The listing builds one solid part. Answer for the finished solid, in the listing's coordinates (mm). A direction names the side the tool comes from. Give positions to 0.01 mm unless a question says otherwise; leave off trailing zeros. Order: outer loops, then holes, each group sorted by start corner. A loop starts at its lowest first (then second) coordinate and runs counter-clockwise, first axis right, second up. Notation, with made-up numbers: M -33.5,72.5 L 15.5,72.5 A26 cw 15.5,88.5 Z; hole C -9.5,73.25 d1. An arc over 180 degrees is marked long. Answer as a JSON object with one key per item and string values. Group by question number.
```python
from build123d import *

# Parameters (mm, degrees)
SKETCH1_R           = 1
SKETCH1_R_2         = 2.25
SKETCH1_R_3         = 1.6
BOSS_EXTRUDE1_DEPTH = 3
SKETCH4_R           = 6.495043718
SKETCH4_R_2         = 4.9
BOSS_EXTRUDE3_DEPTH = 5
SKETCH6_W           = 8.48311055
SKETCH6_H           = 1.891574962
CUT_EXTRUDE3_DEPTH  = 34


with BuildPart() as part:
    # Sketch1 → Boss-Extrude1 (new body)
    with BuildSketch(Plane(origin=(0, 0, 0), x_dir=(1, 0, 0), z_dir=(0, 1, 0))):
        Polygon((43.076410298, 50.123925917), (42.618597625, 48.402115535), (19.4637773, 25.158118275), (-19.4637773, 25.158118275), (-42.618597625, 48.402115535), (-45.64603124, 59.788140743), (-55.300297258, 62.394891143), (-62.384942335, 55.337426715), (-59.815321393, 45.673211889), (-50.185022628, 43.072932893), (-35, 26.288270568), (-34.873, 0), (-35, -26.288270568), (-50.185022628, -43.072932893), (-59.815321393, -45.673211889), (-62.384942335, -55.337426715), (-55.300297258, -62.394891143), (-45.64603124, -59.788140743), (-42.618597625, -48.402115535), (-19.4637773, -25.158118275), (19.4637773, -25.158118275), (42.618597625, -48.402115535), (45.64603124, -59.788140743), (55.300297258, -62.394891143), (62.384942335, -55.337426715), (59.815321393, -45.673211889), (50.185022628, -43.072932893), (35, -26.288270568), (34.873, 0), (35, 26.288270568), (50.185022628, 43.072932893), (59.815321393, 45.673211889), (62.384942335, 55.337426715), (55.300297258, 62.394891143), (45.64603124, 59.788140743), align=None)
        with Locations(Location((-52.730676316, -57.230676316, 0), (0, 0, 270))):
            Circle(SKETCH1_R, mode=Mode.SUBTRACT)
        with Locations(Location((-57.230676316, -52.730676316, 0), (0, 0, 270))):
            Circle(SKETCH1_R, mode=Mode.SUBTRACT)
        with Locations(Location((-48.230676316, -52.730676316, 0), (0, 0, 270))):
            Circle(SKETCH1_R, mode=Mode.SUBTRACT)
        with Locations(Location((-52.730676316, -48.230676316, 0), (0, 0, 270))):
            Circle(SKETCH1_R, mode=Mode.SUBTRACT)
        with Locations(Location((-30, -17, 0), (0, 0, 270))):
            Circle(SKETCH1_R_2, mode=Mode.SUBTRACT)
        with Locations(Location((-15.25, -15.25, 0), (0, 0, 270))):
            Circle(SKETCH1_R_3, mode=Mode.SUBTRACT)
        with Locations(Location((52.730676316, -57.230676316, 0), (0, 0, 270))):
            Circle(SKETCH1_R, mode=Mode.SUBTRACT)
        with Locations(Location((48.230676316, -52.730676316, 0), (0, 0, 270))):
            Circle(SKETCH1_R, mode=Mode.SUBTRACT)
        with Locations(Location((52.730676316, -48.230676316, 0), (0, 0, 270))):
            Circle(SKETCH1_R, mode=Mode.SUBTRACT)
        with Locations(Location((57.230676316, -52.730676316, 0), (0, 0, 270))):
            Circle(SKETCH1_R, mode=Mode.SUBTRACT)
        with Locations(Location((30, -17, 0), (0, 0, 270))):
            Circle(SKETCH1_R_2, mode=Mode.SUBTRACT)
        with Locations(Location((15.25, -15.25, 0), (0, 0, 270))):
            Circle(SKETCH1_R_3, mode=Mode.SUBTRACT)
        with Locations(Location((-15.25, 15.25, 0), (0, 0, 270))):
            Circle(SKETCH1_R_3, mode=Mode.SUBTRACT)
        with Locations(Location((-30, 17, 0), (0, 0, 270))):
            Circle(SKETCH1_R_2, mode=Mode.SUBTRACT)
        with Locations(Location((-57.230676316, 52.730676316, 0), (0, 0, 270))):
            Circle(SKETCH1_R, mode=Mode.SUBTRACT)
        with Locations(Location((-52.730676316, 48.230676316, 0), (0, 0, 270))):
            Circle(SKETCH1_R, mode=Mode.SUBTRACT)
        with Locations(Location((-48.230676316, 52.730676316, 0), (0, 0, 270))):
            Circle(SKETCH1_R, mode=Mode.SUBTRACT)
        with Locations(Location((-52.730676316, 57.230676316, 0), (0, 0, 270))):
            Circle(SKETCH1_R, mode=Mode.SUBTRACT)
        with Locations(Location((15.25, 15.25, 0), (0, 0, 270))):
            Circle(SKETCH1_R_3, mode=Mode.SUBTRACT)
        with Locations(Location((30, 17, 0), (0, 0, 270))):
            Circle(SKETCH1_R_2, mode=Mode.SUBTRACT)
        with Locations(Location((52.730676316, 48.230676316, 0), (0, 0, 270))):
            Circle(SKETCH1_R, mode=Mode.SUBTRACT)
        with Locations(Location((48.230676316, 52.730676316, 0), (0, 0, 270))):
            Circle(SKETCH1_R, mode=Mode.SUBTRACT)
        with Locations(Location((57.230676316, 52.730676316, 0), (0, 0, 270))):
            Circle(SKETCH1_R, mode=Mode.SUBTRACT)
        with Locations(Location((52.730676316, 57.230676316, 0), (0, 0, 270))):
            Circle(SKETCH1_R, mode=Mode.SUBTRACT)
    extrude(amount=BOSS_EXTRUDE1_DEPTH)

    # Sketch4 → Boss-Extrude3 (add)
    with BuildSketch(Plane.XZ):
        with Locations(Location((0, 0, 0), (0, 0, 90))):
            Circle(SKETCH4_R)
        with Locations(Location((0, 0, 0), (0, 0, 270))):
            Circle(SKETCH4_R_2, mode=Mode.SUBTRACT)
    extrude(amount=BOSS_EXTRUDE3_DEPTH)

    # Sketch6 → Cut-Extrude3 (cut)
    with BuildSketch(Plane.XY.offset(35)):
        with Locations((0, -0.945787481)):
            Rectangle(SKETCH6_W, SKETCH6_H)
    extrude(amount=-CUT_EXTRUDE3_DEPTH, mode=Mode.SUBTRACT)


solid = part.part
```
Item 1: Consider probe 1 along Z at (x, y) = (53.5, 2); probe 2 along Y at (x, z) = (19, 1.5); probe 3 along Z at (x, y) = (-16.5, 1.25). Determine where each line is inside the solid, lowest interval first. Write a range as from..to.
Item 2: Section B-B (x = 15.25) is taken. Determine the outline of the cut face in (y, z).
Item 3: Flat-ended cylindrical pins translate along their axes: P1, Ø3.5, axis at x = 15.25, z = -15.25, coming from the -Y side; P2, Ø15.5, axis at x = 0, z = 0, coming from the -Y side; P3, Ø0.6, axis at y = -1, z = 3, coming from the +X side. Find the tip coordinate at first contact, or state that the pin passes through.
Item 4: Section C-C (x = -30) is taken. Determine the outline of the cut face in (y, z).
Item 5: Section A-A (x = 0) is taken. Determine the outline of the cut face in (y, z), and give its area (3 significant figures).
Item 6: Determine the mould class of faces 1 (the cylindrical face through (30.676, 1.479, -14.854)), 2 (the flat face through (0, 3, 4)), 3 (the flat face through (54.933, 1.479, -44.355)) for opening direction X: released by +X, released by -X, zero draft, split by the parting line, or undercut.
Item 7: A tool of negligible diameter and unlimited length cuts with its end or side. For faces 4 (the cylindrical face through (1.472, -2.465, -4.674)), 5 (the flat face through (61.082, 1.479, -50.438)), 6 (the flat face through (31.2, 1.48, -36.94)), 7 (the flat face through (44.111, 1.479, 54.015)), 8 (the flat face through (-54.933, 1.479, 44.355)), from which of +Z, -Z, +X, -X, +Y, -Y can it reach the whole face along a straight path? Write none if from no direction.
Values found:
{
 "1": {"probe 1": "z = -61.91..-57.87, -56.59..-48.87, -47.59..-43.97, 43.97..47.59, 48.87..56.59, 57.87..61.91", "probe 2": "y = 0..3", "probe 3": "z = -25.16..-16.25, -14.25..14.25, 16.25..25.16"},
 "2": {"outline": "M 0,-25.16 L 3,-25.16 L 3,-16.85 L 0,-16.85 Z; M 0,-13.65 L 3,-13.65 L 3,13.65 L 0,13.65 Z; M 0,16.85 L 3,16.85 L 3,25.16 L 0,25.16 Z"},
 "3": {"P1": "stops at y = 0", "P2": "stops at y = -5", "P3": "stops at x = 5.91"},
 "4": {"outline": "M 0,-35.73 L 3,-35.73 L 3,-19.25 L 0,-19.25 Z; M 0,-14.75 L 3,-14.75 L 3,14.75 L 0,14.75 Z; M 0,19.25 L 3,19.25 L 3,35.73 L 0,35.73 Z"},
 "5": {"outline": "M -5,-6.5 L 0,-6.5 L 0,-25.16 L 3,-25.16 L 3,25.16 L 0,25.16 L 0,-4.9 L -5,-4.9 Z; M -5,4.9 L -1.89,4.9 L -1.89,6.5 L -5,6.5 Z", "area": "164 mm^2"},
 "6": {"face 1": "undercut", "face 2": "zero draft", "face 3": "released by +X"},
 "7": {"face 4": "-Y", "face 5": "+X, +Y, -Y", "face 6": "-Z, +Y, -Y", "face 7": "+Z, +Y, -Y", "face 8": "-X, +Y, -Y"}
}
